Check sheet for the modelled part. Datum: model origin and axes. Units: mm. Face numbers are marked on the shaded views. A direction names the side the tool comes from. Give positions to 0.01 mm unless a question says otherwise; leave off trailing zeros. Write each loop counter-clockwise with the first axis right and the second up, starting at its lowest first coordinate (ties: lowest second). Pieces come first, ordered by that corner, then holes. Notation, with made-up numbers: M -36,77.25 L 18,77.25 A24 ccw 18,107.25 Z; hole C -29,-38 d10. An arc over 180 degrees is marked long. One line per item, written item: value. Start each with the question number.
Autodesk Inventor part; units mm, degrees
ref_plane "YZ Plane" through (0, 0, 0) normal (1, 0, 0) x (0, 1, 0)
ref_plane "XZ Plane" through (0, 0, 0) normal (0, 1, 0) x (-1, 0, 0)
ref_plane "XY Plane" through (0, 0, 0) normal (0, 0, 1) x (1, 0, 0)
sketch "Sketch1" plane through (0, 0, 0) normal (0, 1, 0) x (-1, 0, 0)
  line L0 (0, 0) -> (41, 0)
  line L1 (0, 0) -> (41, 0) construction
  line L2 (41, 0) -> (41, -51)
  line L3 (41, -51) -> (3.5, -51)
  line L4 (3.5, -51) -> (3.5, -41.5)
  line L5 (3.5, -41.5) -> (14, -41.5)
  line L6 (14, -41.5) -> (14, -28)
  line L7 (14, -28) -> (0, -28)
  line L8 (0, -28) -> (0, 0)
  dimension "d0" = 41
  dimension "d1" = 0
  dimension "d2" = 51
  dimension "d3" = 90
  dimension "d4" = 37.5
  dimension "d5" = 90
  dimension "d6" = 9.5
  dimension "d7" = 90
  dimension "d8" = 10.5
  dimension "d9" = 13.5
  dimension "d10" = 90
extrude "Extrusion1" add sketch "Sketch1" along normal blind 29
sketch "Sketch2" plane through (-41, 0, 0) normal (0, 0, 1) x (1, 0, 0)
  line L0 (41, 0) -> (0, 0)
  line L1 (41, 0) -> (41, 29)
  line L2 (0, 29) -> (41, 29)
  line L3 (0, 0) -> (0, 29)
  circle A0 centre (17.25, 14.5) radius 8.625
  dimension "d13" = 17.25
  dimension "d14" = 17.25
  dimension "d15" = 14.5
extrude "Extrusion2" cut sketch "Sketch2" against normal blind 3 contours A0
sketch "Sketch3" plane through (-14, 0, -28) normal (1, 0, 0) x (0, 0, -1)
  line L0 (13.5, 0) -> (0, 0)
  line L1 (13.5, 0) -> (13.5, 29)
  line L2 (0, 29) -> (13.5, 29)
  line L3 (0, 0) -> (0, 29)
  line L4 (0, 0) -> (-28, 0)
  line L5 (0, 0) -> (0, 29)
  line L6 (-28, 29) -> (0, 29)
  line L7 (-28, 0) -> (-28, 29)
  line L8 (23, 0) -> (13.5, 0)
  line L9 (23, 0) -> (23, 29)
  line L10 (13.5, 29) -> (23, 29)
  line L11 (13.5, 0) -> (13.5, 29)
  line L12 (2.7351, 24.5) -> (10.7649, 24.5)
  line L13 (10.7649, 24.5) -> (10.7649, 4.5)
  line L14 (10.7649, 4.5) -> (2.7351, 4.5)
  line L15 (2.7351, 4.5) -> (2.7351, 24.5)
  line L16 (2.7351, 24.5) -> (10.7649, 4.5) construction
  line L17 (10.7649, 24.5) -> (2.7351, 4.5) construction
  line L18 (-15.0444, 25.4539) -> (-4.0444, 25.4539)
  line L19 (-4.0444, 25.4539) -> (-4.0444, 3.5461)
  line L20 (-4.0444, 3.5461) -> (-15.0444, 3.5461)
  line L21 (-15.0444, 3.5461) -> (-15.0444, 25.4539)
  line L22 (-15.0444, 25.4539) -> (-4.0444, 3.5461) construction
  line L23 (-4.0444, 25.4539) -> (-15.0444, 3.5461) construction
  line L24 (17.7718, 7.3132) -> (17.7718, 21.6868) construction
  line L25 (20.5552, 7.3132) -> (20.5552, 21.6868)
  line L26 (14.9884, 21.6868) -> (14.9884, 7.3132)
  arc A0 (14.9884, 7.3132) -> (20.5552, 7.3132) centre (17.7718, 7.3132) ccw
  arc A1 (20.5552, 21.6868) -> (14.9884, 21.6868) centre (17.7718, 21.6868) ccw
  point P0 (6.75, 14.5)
  point P1 (-9.5444, 14.5)
  point P2 (17.7718, 14.5)
  dimension "d18" = 20
  dimension "d19" = 11
extrude "Extrusion3" add sketch "Sketch3" along normal blind 19 contours L12 L13 L14 L15 | L18 L19 L20 L21 | A0 L26 A1 L25
ref_plane "Work Plane1" through (-23.75, 14.5, -3) normal (0, 1, 0) x (1, 0, 0)
properties part number "00_RGB_Laser_Laserlands"
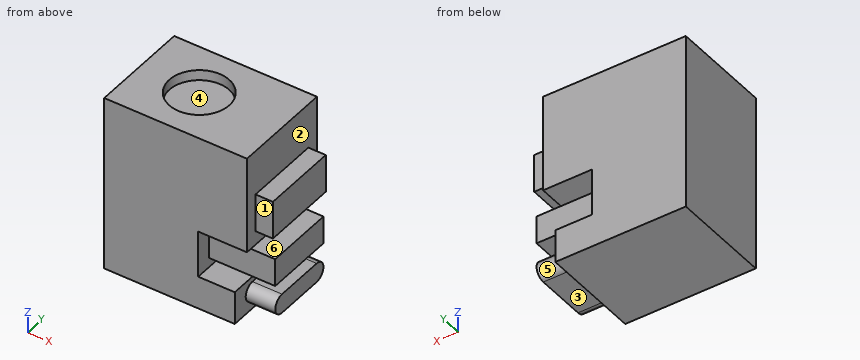
1) Cross-section at A-A (y = 2.25). Record the boundary of the cut face in (x, z).
2) Gauge pin test, flat ends, axial feed: pin 1 (5 mm diameter, centred on x = -11.5, y = 10.5, fed in from +Z); pin 2 (2.5 mm diameter, centred on x = 3, y = 17.5, fed in from -Z); pin 3 (8.5 mm diameter, centred on x = -23.5, y = 14.5, fed in from +Z); pin 4 (2.5 mm diameter, centred on x = 2.5, z = -17, fed in from -Y). Record the tip position at first contact, or that the pin passes through.
3) Cross-section at C-C (x = 1.5). Record the boundary of the cut face in (y, z), plus the area to 3 significant figures.
4) Cross-section at D-D (z = -25). Record the boundary of the cut face in (x, y), plus the area to 3 significant figures.
5) Draft check along Z on the marked faces 1, 2 and 3. Enter one of: released by +Z, released by -Z, zero draft, split by the parting line, or undercut.
6) Material ranges on L1, parallel to Z at x = -8.5, y = 20; L2, parallel to Z at x = -3, y = 14.5; L3, parallel to X at y = 6.75, z = -10, recorded low to high. Write a range as from..to.
7) Cross-section at B-B (x = -23.75). Record the boundary of the cut face in (y, z) (3 decimals), plus the area to 3 significant figures.
8) Tool access check on the marked faces 4, 5 and 6. Record the directions out of +Z, -Z, +X, -X, +Y, -Y that give a thin tool (end or side, any length) a straight path to the whole face; none if there is none.
Data:
1. outline: M -41,-51 L -3.5,-51 L -3.5,-41.5 L -14,-41.5 L -14,-28 L 0,-28 L 0,0 L -41,0 Z
2. pin 1: stops at z = 0
2. pin 2: stops at z = -48.56
2. pin 3: stops at z = -3
2. pin 4: stops at y = 3.55
3. outline: M 3.55,-23.96 L 25.45,-23.96 L 25.45,-12.96 L 3.55,-12.96 Z; M 4.5,-38.76 L 24.5,-38.76 L 24.5,-30.74 L 4.5,-30.74 Z; M 7.31,-48.56 L 21.69,-48.56 A2.78 ccw 21.69,-42.99 L 7.31,-42.99 A2.78 ccw Z
3. area: 506 mm2
4. outline: M -41,0 L 0,0 L 0,29 L -41,29 Z
4. area: 1,190 mm2
5. face 1: zero draft
5. face 2: undercut
5. face 3: released by -Z
6. L1: z = -51..-41.5, -38.76..-30.74, -28..0
6. L2: z = -48.56..-42.99, -38.76..-30.74, -28..0
6. L3: x = -41..0
7. outline: M 0,-51 L 29,-51 L 29,0 L 23.125,0 L 23.125,-3 L 5.875,-3 L 5.875,0 L 0,0 Z
7. area: 1,430 mm2
8. face 4: +Z
8. face 5: +X, +Y
8. face 6: +X, +Y, -Y
